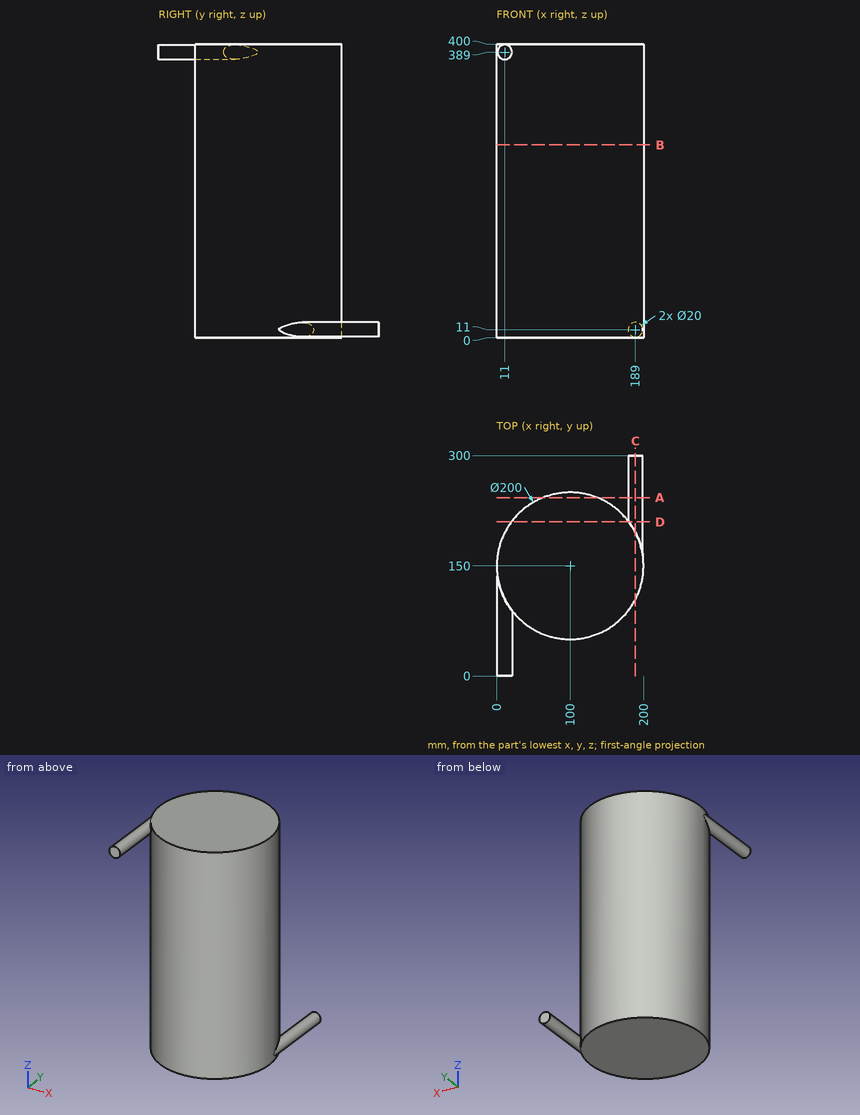
Design review of the part shown in the three views and the two pictorial views. Dimensions are in mm from the part's minimum x, y and z. Coordinates: 2 decimals unless noted, no trailing zeros. Order: outer loops, then holes, each group sorted by start corner. A loop starts at its lowest first (then second) coordinate and runs counter-clockwise, first axis right, second up.
1) Take a section at C-C, the plane x = 189. Give the boundary of the cut face in (y, z).
2) Take a section at B-B, the plane z = 262.5. Give the boundary of the cut face in (x, y), and give its area (3 significant figures).
3) Wall thickness on line 1 along Y through (x, z) = (96, 190); line 2 along Z through (x, y) = (11, 95); line 3 along Y through (x, z) = (118.5, 318): over which ranges is each line inside the solid? List them lowest first.
4) Take a section at D-D, the plane y = 210. Give the boundary of the cut face in (x, z), and give its area (3 significant figures).
5) Clearance check with flat-ended pins moving along their axes: pin 1 (10 mm diameter, centred on y = 217.5, z = 80.5, fed in from +X); pin 2 (2 mm diameter, centred on y = 200, z = 151, fed in from +X); pin 3 (4 mm diameter, centred on y = 169.5, z = 103.5, fed in from -X). State where each tip first meets the part, or that it passes through.
6) Take a section at A-A, the plane y = 243. Give the boundary of the cut face in (x, z).
Returned:
1. outline: (104.4, 0) - (195.6, 0) - (195.6, 1) - (300, 1) - (300, 21) - (195.6, 21) - (195.6, 400) - (104.4, 400) - close
2. outline: circle Ø200 at (100, 150)
2. area: 31,400 mm2
3. line 1: y = 50.08 to 249.92
3. line 2: z = 379 to 399
3. line 3: y = 51.73 to 248.27
4. outline: (20, 0) - (180, 0) - (180, 6.64) arc R10 ccw (long way) to (180, 15.36) - (180, 400) - (20, 400) - close
4. area: 64,300 mm2
5. pin 1: stops at x = 178.06
5. pin 2: stops at x = 187.17
5. pin 3: stops at x = 1.54
6. outline: (63.24, 0) - (136.76, 0) - (136.76, 400) - (63.24, 400) - close; circle Ø20 at (189, 11)
